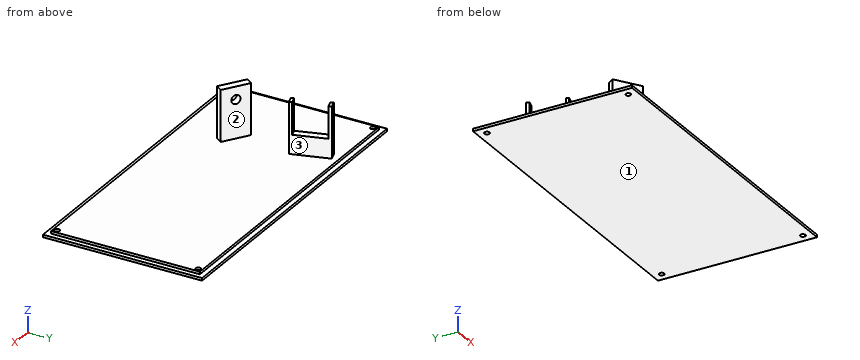
from build123d import *

# Parameters (mm, degrees)
SKIZZE1_W                       = 250
SKIZZE1_H                       = 125
AUFSATZ_LINEAR_AUSTRAGEN1_DEPTH = 2
SKIZZE2_W                       = 242
SKIZZE2_H                       = 117
AUFSATZ_LINEAR_AUSTRAGEN2_DEPTH = 2
SKIZZE3_R                       = 2
SCHNITT_LINEAR_AUSTRAGEN1_DEPTH = 32
AUFSATZ_LINEAR_AUSTRAGEN3_DEPTH = 40
SCHNITT_LINEAR_AUSTRAGEN2_DEPTH = 25
SKIZZE8_R                       = 1
SCHNITT_LINEAR_AUSTRAGEN3_DEPTH = 40
SKIZZE9_R                       = 3.493135661
SCHNITT_LINEAR_AUSTRAGEN4_DEPTH = 20


with BuildPart() as part:
    # Skizze1 → Aufsatz-Linear austragen1 (new body)
    with BuildSketch(Plane.XY):
        with Locations((125, 62.5)):
            Rectangle(SKIZZE1_W, SKIZZE1_H)
    extrude(amount=AUFSATZ_LINEAR_AUSTRAGEN1_DEPTH)

    # Skizze2 → Aufsatz-Linear austragen2 (add)
    with BuildSketch(Plane.XY.offset(2)):
        with Locations((125, 62.5)):
            Rectangle(SKIZZE2_W, SKIZZE2_H)
    extrude(amount=AUFSATZ_LINEAR_AUSTRAGEN2_DEPTH)

    # Skizze3 → Schnitt-Linear austragen1 (cut)
    with BuildSketch(Plane.XY.offset(4)):
        with Locations((7, 118)):
            Circle(SKIZZE3_R)
        with Locations((7, 7)):
            Circle(SKIZZE3_R)
        with Locations((243, 7)):
            Circle(SKIZZE3_R)
        with Locations((243, 118)):
            Circle(SKIZZE3_R)
    extrude(amount=-SCHNITT_LINEAR_AUSTRAGEN1_DEPTH, mode=Mode.SUBTRACT)

    # Skizze4 → Aufsatz-Linear austragen3 (add)
    with BuildSketch(Plane.XY.offset(4)):
        Polygon((62.595258591, 85.778313546), (68.333087126, 87.532543775), (59.561935985, 116.221686454), (53.824107449, 114.467456225), align=None)
        Polygon((54.200560001, 46.732563956), (73.26842417, 33.871127177), (76.623581591, 38.845352612), (57.555717422, 51.706789392), align=None)
    extrude(amount=AUFSATZ_LINEAR_AUSTRAGEN3_DEPTH)

    # Skizze7 → Schnitt-Linear austragen2 (cut)
    with BuildSketch(Plane.XY.offset(44)):
        Polygon((54.49656237, 112.267955287), (60.234390906, 114.022185515), (67.660632206, 89.732044713), (61.92280367, 87.977814485), align=None)
    extrude(amount=-SCHNITT_LINEAR_AUSTRAGEN2_DEPTH, mode=Mode.SUBTRACT)

    # Skizze8 → Schnitt-Linear austragen3 (cut)
    with BuildSketch(Plane(origin=(-27.403744567, 89.633609675, 0), x_dir=(0.9563047559630352, 0.2923717047227376, 0), z_dir=(-0.29237170472273766, 0.9563047559630353, 0))):
        with Locations(Location((87.939295251, -34, 0), (0, 0, 180))):
            Circle(SKIZZE8_R)
    extrude(amount=-SCHNITT_LINEAR_AUSTRAGEN3_DEPTH, mode=Mode.SUBTRACT)

    # Skizze9 → Schnitt-Linear austragen4 (cut)
    with BuildSketch(Plane(origin=(41.968333241, 62.220612777, 0), x_dir=(0.8290375725550413, -0.5591929034707476, 0), z_dir=(0.5591929034707476, 0.8290375725550413, 0))):
        with Locations(Location((30.301782569, -34, 0), (0, 0, 180))):
            Circle(SKIZZE9_R)
    extrude(amount=-SCHNITT_LINEAR_AUSTRAGEN4_DEPTH, mode=Mode.SUBTRACT)


solid = part.part
Geometry check sheet. Reference: the model listing, model coordinates, mm. Face numbers are marked on the shaded views. Coordinates: 2 decimals unless noted, no trailing zeros. Order: outer loops, then holes, each group sorted by start corner. A loop starts at its lowest first (then second) coordinate and runs counter-clockwise, first axis right, second up. Notation, with made-up numbers: M 4.25,87 L 30.25,87 A16 ccw 30.25,93 Z; hole C 48.5,51.5 d10. An arc over 180 degrees is marked long. Use CSV: the item, a comma, the result in double quotes.
Item 1: Thickness scan on line 1 along Y through (x, z) = (243, 2.9); line 2 along Y through (x, z) = (243, 1); line 3 along Z through (x, y) = (149.5, 10). Record the ranges inside material, lowest first.
Returned:
line 1,"y = 4 to 5, 9 to 116, 120 to 121"
line 2,"y = 0 to 5, 9 to 116, 120 to 125"
line 3,"z = 0 to 4"
Item 2: Cross-section at D-D on z = 14. Record the cut outline in (x, y).
Returned:
outline,"M 53.82,114.47 L 62.6,85.78 L 68.33,87.53 L 59.56,116.22 Z; M 54.2,46.73 L 73.27,33.87 L 76.62,38.85 L 57.56,51.71 Z"
Item 3: Cross-section at B-B on x = 227. Record the cut outline in (y, z), then the cut area to 3 significant figures.
Returned:
outline,"M 0,0 L 125,0 L 125,2 L 121,2 L 121,4 L 4,4 L 4,2 L 0,2 Z"
area,"484 mm2"
Item 4: Cross-section at C-C on y = 68. Record the cut outline in (x, z), then the cut area to 3 significant figures.
Returned:
outline,"M 0,0 L 250,0 L 250,2 L 246,2 L 246,4 L 4,4 L 4,2 L 0,2 Z"
area,"984 mm2"
Item 5: Mould release check, pull along Y, two halves, no side actions. Record for the marked faces 1, 2 and 3: pulls with the +Y half, pulls with the -Y half, needs draft (parallel to the pull), parting line crosses it, or undercut.
Returned:
face 1,"needs draft"
face 2,"undercut"
face 3,"pulls with the +Y half"
Item 6: Gauge pin test, flat ends, axial feed: pin 1 Ø12 at (x, y) = (28.5, 61.5) entering from +Z; pin 2 Ø3 at (x, y) = (7, 118) entering from +Z (3 decimals); pin 3 Ø6.5 at (x, y) = (60, 105.5) entering from +Z; pin 4 Ø1.6 at (y, z) = (62, 3) entering from -X. Record the tip position at first contact, or that the pin passes through.
Returned:
pin 1,"stops at z = 4"
pin 2,"passes through"
pin 3,"stops at z = 19"
pin 4,"stops at x = 4"
Item 7: Cross-section at A-A on z = 25. Record the cut outline in (x, y).
Returned:
outline,"M 53.82,114.47 L 54.5,112.27 L 60.23,114.02 L 59.56,116.22 Z; M 54.2,46.73 L 73.27,33.87 L 76.62,38.85 L 57.56,51.71 Z; M 61.92,87.98 L 62.6,85.78 L 68.33,87.53 L 67.66,89.73 Z"
